Read the model definition and answer for the solid it produces. Units are mm, in the model's axes. A direction names the side the tool comes from. Coordinates: 2 decimals unless noted, no trailing zeros. Order: outer loops, then holes, each group sorted by start corner. A loop starts at its lowest first (then second) coordinate and runs counter-clockwise, first axis right, second up. Notation, with made-up numbers: (61.5, -34.75) -> (113.5, -34.75) arc R13 cw to (113.5, -27.75) -> close; hole circle Ø1 at (59, 36). An arc over 180 degrees is marked (long way). Answer as a JSON object with one key per item and string values. Group by question number.
1) Given pin 1 (19 mm diameter, centred on y = -46.5, z = 93.5, fed in from +X); pin 2 (12.5 mm diameter, centred on x = 6.5, y = -31.5, fed in from +Z); pin 3 (4 mm diameter, centred on y = -7, z = 95.5, fed in from -X) (3 decimals), each flat-ended and moving along its own axis, determine where each tip first touches the part or whether it passes through.
2) A tool of negligible diameter and unlimited length cuts with its end or side. For faces 4 (the flat face through (15.875, -32, 69)), 5 (the flat face through (96, -31, 12.7)), 6 (the flat face through (54, -31, 12.7)), from which of +Z, -Z, +X, -X, +Y, -Y can it reach the whole face along a straight path? Write none if from no direction.
3) Section C-C on x = 73 is taken. Determine the outline of the cut face in (y, z), and give its area (3 significant figures).
4) Determine the mould class of faces 1 (the cylindrical face through (92.116, -31.364, 105.565)), 2 (the flat face through (19.05, -31, 69)), 3 (the flat face through (49, 0, 11)) for opening direction Y: released by +Y, released by -Y, zero draft, split by the parting line, or undercut.
5) Section B-B on y = -24 is taken. Determine the outline of the cut face in (x, z) (3 decimals).
6) Section A-A on z = 104 is taken. Determine the outline of the cut face in (x, y) (3 decimals), and give its area (3 significant figures).
7) Consider L1, parallel to X at y = -17, z = 18.5 (3 decimals); L2, parallel to Z at x = 45.5, y = -18.5. Determine where each line is inside the solid, lowest interval first.
Autodesk Inventor part; units mm, degrees
ref_plane "YZ Plane" through (0, 0, 0) normal (1, 0, 0) x (0, 1, 0)
ref_plane "XZ Plane" through (0, 0, 0) normal (0, 1, 0) x (-1, 0, 0)
ref_plane "XY Plane" through (0, 0, 0) normal (0, 0, 1) x (1, 0, 0)
sketch "Sketch1" plane through (0, 0, 0) normal (0, 0, 1) x (1, 0, 0)
  line L0 (0, 0) -> (98.171, 0)
  line L1 (98.171, 0) -> (98.171, -63.5)
  line L2 (98.171, -63.5) -> (0, -63.5)
  line L3 (0, -63.5) -> (0, 0)
  dimension "d0" = 98.171
  dimension "d1" = 63.5
extrude "Extrusion1" add sketch "Sketch1" along normal blind 12.7
sketch "Sketch2" plane through (0, 0, 12.7) normal (0, 0, 1) x (1, 0, 0)
  line L0 (0, -63.5) -> (98.171, -63.5)
  line L1 (98.171, -63.5) -> (90.551, -63.5)
  line L2 (90.551, -63.5) -> (93.726, -63.5)
  line L3 (93.726, -63.5) -> (93.726, 0)
  line L4 (93.726, 0) -> (90.551, 0)
  line L5 (90.551, 0) -> (90.551, -63.5)
  point P0 (0, 0)
  dimension "d4" = 7.62
  dimension "d5" = 3.175
extrude "Extrusion2" add sketch "Sketch2" along normal blind 114.3
sketch "Sketch3" plane through (0, 0, 12.7) normal (0, 0, 1) x (1, 0, 0)
  line L0 (0, 0) -> (15.875, 0)
  line L1 (90.551, 0) -> (0, 0)
  line L2 (0, -63.5) -> (90.551, -63.5)
  line L3 (15.875, 0) -> (19.05, 0)
  line L4 (19.05, 0) -> (19.05, -63.5)
  line L5 (19.05, -63.5) -> (15.875, -63.5)
  line L6 (15.875, -63.5) -> (15.875, 0)
  dimension "d8" = 15.875
  dimension "d9" = 3.175
extrude "Extrusion3" add sketch "Sketch3" along normal blind 114.3
sketch "Sketch4" plane through (15.875, -63.5, 12.7) normal (-1, 0, 0) x (0, 0, 1)
  circle A0 centre (95.8596, 32.004) radius 2.9972
  point P0 (-12.7, 63.5)
  point P1 (114.3, 63.5)
  dimension "d14" = 5.9944
extrude "Extrusion4" cut sketch "Sketch4" against normal blind 101.6
properties part number "ChainWheelSubAssemblyMainConnector"
Worked answers:
{
 "1": {"pin 1": "stops at x = 93.73", "pin 2": "stops at z = 12.7", "pin 3": "stops at x = 15.875"},
 "2": {"face 4": "+Z, -X, +Y, -Y", "face 5": "+Z, +X, +Y, -Y", "face 6": "+Z, +Y, -Y"},
 "3": {"outline": "(-63.5, 0) -> (0, 0) -> (0, 12.7) -> (-63.5, 12.7) -> close", "area": "806 mm²"},
 "4": {"face 1": "undercut", "face 2": "zero draft", "face 3": "released by +Y"},
 "5": {"outline": "(0, 0) -> (98.171, 0) -> (98.171, 12.7) -> (93.726, 12.7) -> (93.726, 127) -> (90.551, 127) -> (90.551, 12.7) -> (19.05, 12.7) -> (19.05, 127) -> (15.875, 127) -> (15.875, 12.7) -> (0, 12.7) -> close"},
 "6": {"outline": "(15.875, -63.5) -> (19.05, -63.5) -> (19.05, 0) -> (15.875, 0) -> close; (90.551, -63.5) -> (93.726, -63.5) -> (93.726, 0) -> (90.551, 0) -> close", "area": "403 mm²"},
 "7": {"L1": "x = 15.875 to 19.05, 90.551 to 93.726", "L2": "z = 0 to 12.7"}
}
